from build123d import *

# Parameters (mm, degrees)
CROQUIS1_W              = 15
CROQUIS1_H              = 5
SALIENTE_EXTRUIR1_DEPTH = 90
SALIENTE_EXTRUIR2_DEPTH = 5
CROQUIS3_W              = 23
CROQUIS3_H              = 7.5
CROQUIS3_H_2            = 5
SALIENTE_EXTRUIR3_DEPTH = 5


with BuildPart() as part:
    # Croquis1 → Saliente-Extruir1 (new body)
    with BuildSketch(Plane.XY):
        Rectangle(CROQUIS1_W, CROQUIS1_H)
    extrude(amount=SALIENTE_EXTRUIR1_DEPTH)

    # Croquis2 → Saliente-Extruir2 (add)
    with BuildSketch(Plane(origin=(0, 0, 0), x_dir=(-1, 0, 0), z_dir=(0, 0, -1))):
        Polygon((-7.5, 2.5), (-15.5, 2.5), (-15.5, -2.5), (-7.5, -2.5), (7.5, -2.5), (7.5, 2.5), align=None)
    extrude(amount=SALIENTE_EXTRUIR2_DEPTH)

    # Croquis3 → Saliente-Extruir3 (add)
    with BuildSketch(Plane(origin=(0, 2.5, 0), x_dir=(1, 0, 0), z_dir=(0, 1, 0))):
        with Locations((4, -8.75)):
            Rectangle(CROQUIS3_W, CROQUIS3_H)
        with Locations((4, -82.5)):
            Rectangle(CROQUIS3_W, CROQUIS3_H_2)
    extrude(amount=-SALIENTE_EXTRUIR3_DEPTH)


solid = part.part
Input: part model. Units: mm. Frame: model coordinates. A direction names the side the tool comes from. Coordinates: 2 decimals unless noted, no trailing zeros. Loops run counter-clockwise (first coordinate to the right, second up) from the corner with the lowest first, then second, coordinate; pieces in that order, holes last.
Q1. Cut plane B-B (y = -1.1). Output: boundary loops of the cut face in (x, z), then the cut area to 4 significant figures.
Q2. Draft query along Z for faces 1 (the face through (4, 0, -5)), 2 (the face through (7.5, 0, 2)), 3 (the face through (11, 0, 12.5)), 4 (the face through (15.5, 0, 83)). Return one class per face: +Z half, -Z half, draft (parallel to the pull), parting line (faces both ways), or undercut.
Q3. Cut plane C-C (z = 69). Output: boundary loops of the cut face in (x, y), then the cut area to 3 significant figures.
Q4. Material intervals for line 1 (Z direction, x = 9, y = 0.65); line 2 (X direction, y = -1.65, z = 70), sorted ascending.
Q5. Contact query for flat-ended pins moving along their axis: pin 1 (2.5 mm diameter, centred on x = 10.5, y = -1, fed in from +Z); pin 2 (1.5 mm diameter, centred on y = 1, z = 2, fed in from +X). Output: stop coordinate, or through.
Q6. Cut plane A-A (x = 10.75). Output: boundary loops of the cut face in (y, z), then the cut area to 3 significant figures.
Q7. Set-up query: faces 5 (the face through (7.5, 0, 87)), 6 (the face through (11, 0, 80)), 7 (the face through (-7.5, 0, 43)). Return all of +Z, -Z, +X, -X, +Y, -Y with unobstructed straight access to the full face (end or side cutting, diameter ignored); none if empty.
Working result:
1. outline: (-7.5, -5) - (15.5, -5) - (15.5, 0) - (7.5, 0) - (7.5, 5) - (15.5, 5) - (15.5, 12.5) - (7.5, 12.5) - (7.5, 80) - (15.5, 80) - (15.5, 85) - (7.5, 85) - (7.5, 90) - (-7.5, 90) - close
1. area: 1,565 mm2
2. face 1: -Z half
2. face 2: undercut
2. face 3: undercut
2. face 4: draft
3. outline: (-7.5, -2.5) - (7.5, -2.5) - (7.5, 2.5) - (-7.5, 2.5) - close
3. area: 75.0 mm2
4. line 1: z = -5 to 0, 5 to 12.5, 80 to 85
4. line 2: x = -7.5 to 7.5
5. pin 1: stops at z = 85
5. pin 2: stops at x = 7.5
6. outline: (-2.5, -5) - (2.5, -5) - (2.5, 0) - (-2.5, 0) - close; (-2.5, 5) - (2.5, 5) - (2.5, 12.5) - (-2.5, 12.5) - close; (-2.5, 80) - (2.5, 80) - (2.5, 85) - (-2.5, 85) - close
6. area: 87.5 mm2
7. face 5: +Z, +X, +Y, -Y
7. face 6: +X, +Y, -Y
7. face 7: +Z, -Z, -X, +Y, -Y
